```python
from build123d import *

# Parameters (mm, degrees)
CHAMFER1_SIZE = 0.127


with BuildPart() as part:
    # Sketch1 → Revolve1 (revolve)
    with BuildSketch(Plane.XY, mode=Mode.PRIVATE) as revolve1_sk:
        Polygon((2.4892, 4.7752), (2.4892, 0), (34.925, 0), (34.925, 2.38125), (31.75, 2.38125), (31.75, 89.69375), (34.925, 89.69375), (34.925, 92.075), (2.4892, 92.075), (2.4892, 46.0375), (2.4892, 36.4998), align=None)
    revolve(revolve1_sk.sketch.rotate(Axis((0, 92.075, 0), (0, -1, 0)), 180), axis=Axis((0, 92.075, 0), (0, -1, 0)))

    # Chamfer1
    chamfer1_edges = [part.edges().sort_by_distance(p)[0] for p in [
        (34.925, 2.38125, 0),
        (34.925, 0, 0),
        (2.4892, 0, 0),
        (2.4892, 92.075, 0),
        (34.925, 92.075, 0),
        (34.925, 89.69375, 0),
    ]]
    chamfer(chamfer1_edges, length=CHAMFER1_SIZE)


solid = part.part
```
The listing builds one solid part. Answer for the finished solid, in the listing's coordinates (mm). A direction names the side the tool comes from. Coordinates: 2 decimals unless noted, no trailing zeros. Loops run counter-clockwise (first coordinate to the right, second up) from the corner with the lowest first, then second, coordinate; pieces in that order, holes last. Notation, with made-up numbers: (17.25, 77.25) -> (28.25, 77.25) arc R8 cw to (28.25, 84.25) -> close; hole circle Ø10 at (44.25, 23). An arc over 180 degrees is marked (long way). Return JSON: item names as keys, results as strings. Group by question number.
(1) Which of the six approach directions +Z, -Z, +X, -X, +Y, -Y give full straight-line access (tool end or side, diameter ignored) to faces 4 (the flat face through (0, 92.075, 7)), 5 (the flat face through (-8, 89.694, 31))?
(2) A cutting plane is placed at C-C on y = 41.5. Write down the section's boundary in (x, z).
(3) Determine the mould class of faces 1 (the cylindrical face through (-2.374, 45.395, -0.748)), 2 (the flat face through (8, 2.381, 31)), 3 (the flat face through (0, 0, 7)) for opening direction Y: released by +Y, released by -Y, zero draft, split by the parting line, or undercut.
(4) Given pin 1 Ø6 at (x, y) = (-13, 45) entering from -Z; pin 2 Ø6 at (x, y) = (-14, 51.5) entering from -Z; pin 3 Ø6 at (y, z) = (61.5, 18) entering from -X; pin 4 Ø8 at (x, z) = (0, 0) entering from +Y (3 decimals), each flat-ended and moving along its own axis, determine where each tip first touches the part or whether it passes through.
(5) Find the intervals of material crossed by probe 1 along Z at (x, y) = (0, 36.5); probe 2 along Y at (x, z) = (-23.5, -23) (3 decimals); probe 3 along X at (y, z) = (42.5, -24.5), in increasing order. Write a range as from..to.
(6) A cutting plane is placed at B-B on z = 0. Write down the section's boundary in (x, y) (3 decimals), and give its area (3 significant figures).
(7) A cutting plane is placed at A-A on x = 0. Write down the section's boundary in (y, z) (3 decimals).
The answers:
{
 "1": {"face 4": "+Z, -Z, +X, -X, +Y", "face 5": "none"},
 "2": {"outline": "circle Ø63.5 at (0, 0); hole circle Ø4.98 at (0, 0)"},
 "3": {"face 1": "zero draft", "face 2": "undercut", "face 3": "released by -Y"},
 "4": {"pin 1": "stops at z = -30.13", "pin 2": "stops at z = -29.78", "pin 3": "stops at x = -27.98", "pin 4": "stops at y = 92.075"},
 "5": {"probe 1": "z = -31.75..-2.49, 2.49..31.75", "probe 2": "y = 0..2.381, 89.694..92.075", "probe 3": "x = -20.19..20.19"},
 "6": {"outline": "(-34.925, 0.127) -> (-34.798, 0) -> (-2.616, 0) -> (-2.489, 0.127) -> (-2.489, 91.948) -> (-2.616, 92.075) -> (-34.798, 92.075) -> (-34.925, 91.948) -> (-34.925, 89.821) -> (-34.798, 89.694) -> (-31.75, 89.694) -> (-31.75, 2.381) -> (-34.798, 2.381) -> (-34.925, 2.254) -> close; (2.489, 0.127) -> (2.616, 0) -> (34.798, 0) -> (34.925, 0.127) -> (34.925, 2.254) -> (34.798, 2.381) -> (31.75, 2.381) -> (31.75, 89.694) -> (34.798, 89.694) -> (34.925, 89.821) -> (34.925, 91.948) -> (34.798, 92.075) -> (2.616, 92.075) -> (2.489, 91.948) -> close", "area": "5,420 mm^2"},
 "7": {"outline": "(0, -34.798) -> (0.127, -34.925) -> (2.254, -34.925) -> (2.381, -34.798) -> (2.381, -31.75) -> (89.694, -31.75) -> (89.694, -34.798) -> (89.821, -34.925) -> (91.948, -34.925) -> (92.075, -34.798) -> (92.075, -2.616) -> (91.948, -2.489) -> (0.127, -2.489) -> (0, -2.616) -> close; (0, 2.616) -> (0.127, 2.489) -> (91.948, 2.489) -> (92.075, 2.616) -> (92.075, 34.798) -> (91.948, 34.925) -> (89.821, 34.925) -> (89.694, 34.798) -> (89.694, 31.75) -> (2.381, 31.75) -> (2.381, 34.798) -> (2.254, 34.925) -> (0.127, 34.925) -> (0, 34.798) -> close"}
}
